```python
from build123d import *

# Parameters (mm, degrees)
F0_W     = 25.4
F0_H     = 6.35
F1_DEPTH = 6.35
F3_DEPTH = 25.4
F4_R     = 0.254
F5_R     = 0.254


with BuildPart() as f1:
    # F0 (on Top) → F1 (new body)
    with BuildSketch(Plane.XY):
        with Locations((12.7, 3.175)):
            Rectangle(F0_W, F0_H)
    extrude(amount=F1_DEPTH)

    # F2 (on face) → F3 (cut)
    with BuildSketch(Plane.XY.offset(6.35)):
        Polygon((15.621, 6.35), (12.7, 6.35), (14.1664696837, 3.81), (15.6269696837, 6.3396602045), align=None)
        Polygon((15.6329393675, 6.35), (15.621, 6.35), (15.6269696837, 6.3396602045), align=None)
        Polygon((15.6329393675, 6.35), (15.6269696837, 6.3396602045), (17.0874696837, 3.81), (18.5479696837, 6.3396602045), (18.542, 6.35), align=None)
        Polygon((18.5539393675, 6.35), (18.542, 6.35), (18.5479696837, 6.3396602045), align=None)
        Polygon((18.5539393675, 6.35), (18.5479696837, 6.3396602045), (20.0084696837, 3.81), (21.4689696837, 6.3396602045), (21.463, 6.35), align=None)
        Polygon((21.4749393675, 6.35), (21.463, 6.35), (21.4689696837, 6.3396602045), align=None)
        Polygon((21.4749393675, 6.35), (21.4689696837, 6.3396602045), (22.9294696837, 3.81), (24.3959393675, 6.35), align=None)
    extrude(amount=-F3_DEPTH, mode=Mode.SUBTRACT)

    # F4
    f4_edges = [f1.edges().sort_by_distance(p)[0] for p in [
        (21.46897, 6.33966, 3.175),
    ]]
    fillet(f4_edges, radius=F4_R)

    # F5
    f5_edges = [f1.edges().sort_by_distance(p)[0] for p in [
        (24.395939, 6.35, 3.175),
        (22.92947, 3.81, 3.175),
        (20.00847, 3.81, 3.175),
        (18.54797, 6.33966, 3.175),
        (17.08747, 3.81, 3.175),
        (15.62697, 6.33966, 3.175),
        (14.16647, 3.81, 3.175),
    ]]
    fillet(f5_edges, radius=F5_R)


solid = f1.part
```
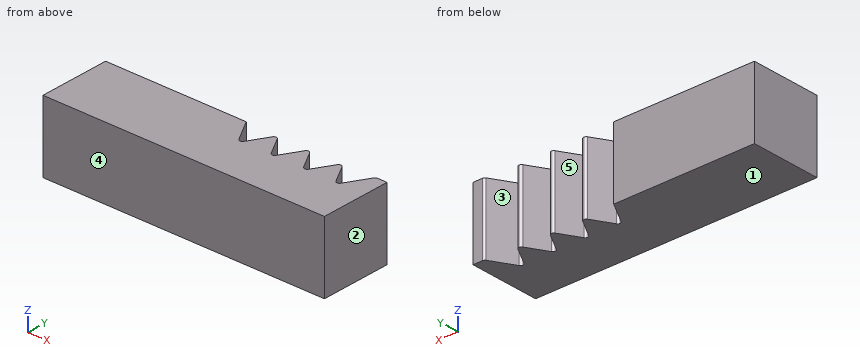
The listing builds one solid part. Answer for the finished solid, in the listing's coordinates (mm). Face numbers are marked on the shaded views. A direction names the side the tool comes from. Give positions to 0.01 mm unless a question says otherwise; leave off trailing zeros. Order: outer loops, then holes, each group sorted by start corner. A loop starts at its lowest first (then second) coordinate and runs counter-clockwise, first axis right, second up. Notation, with made-up numbers: (89, 62.25) -> (93, 62.25) arc R31 cw to (93, 97.25) -> close; hole circle Ø11 at (67, -31). An arc over 180 degrees is marked (long way). Answer as CSV lines item,"result". Start each with the question number.
Q1. Given pin 1 (1.5 mm diameter, centred on x = 2.5, y = 3, fed in from -Z), flat-ended and moving along its own axis, determine where the tip first touches the part or whether it passes through.
Q2. Which of the six approach directions +Z, -Z, +X, -X, +Y, -Y give full straight-line access (tool end or side, diameter ignored) to the marked faces 4 and 5?
Q3. A cutting plane is placed at C-C (x = 23.5). Determine the outline of the cut face in (y, z), then the cut area to 3 significant figures.
Q4. A cutting plane is placed at D-D (y = 4.5). Determine the outline of the cut face in (x, z).
Q5. Determine the mould class of the marked faces 1, 2 and 3 for opening direction X: pulls with the +X half, pulls with the -X half, needs draft (parallel to the pull), parting line crosses it, or undercut.
Q6. A cutting plane is placed at A-A (z = 1.5). Determine the outline of the cut face in (x, y).
Q7. A cutting plane is placed at B-B (y = 5.5). Determine the outline of the cut face in (x, z), then the cut area to 3 significant figures.
Q8. Find the intervals of material crossed by L1, parallel to X at y = 5, z = 1.75; L2, parallel to X at y = 5.25, z = 1.25; L3, parallel to X at y = 6.25, z = 5.5, in increasing order.
Results found:
1,pin 1,"z = 0"
2,face 4,"+Z, -Z, +X, -X, -Y"
2,face 5,"+Z, -Z, +Y"
3,outline,"(0, 0) -> (4.8, 0) -> (4.8, 6.35) -> (0, 6.35) -> close"
3,area,"30.5 mm2"
4,outline,"(0, 0) -> (13.77, 0) -> (13.77, 6.35) -> (0, 6.35) -> close; (14.56, 0) -> (16.69, 0) -> (16.69, 6.35) -> (14.56, 6.35) -> close; (17.49, 0) -> (19.61, 0) -> (19.61, 6.35) -> (17.49, 6.35) -> close; (20.41, 0) -> (22.53, 0) -> (22.53, 6.35) -> (20.41, 6.35) -> close; (23.33, 0) -> (25.4, 0) -> (25.4, 6.35) -> (23.33, 6.35) -> close"
5,face 1,"needs draft"
5,face 2,"pulls with the +X half"
5,face 3,"undercut"
6,outline,"(0, 0) -> (25.4, 0) -> (25.4, 6.35) -> (24.54, 6.35) arc R0.25 ccw to (24.32, 6.22) -> (23.15, 4.19) arc R0.25 cw to (22.71, 4.19) -> (21.69, 5.96) arc R0.25 ccw to (21.25, 5.96) -> (20.23, 4.19) arc R0.25 cw to (19.79, 4.19) -> (18.77, 5.96) arc R0.25 ccw to (18.33, 5.96) -> (17.31, 4.19) arc R0.25 cw to (16.87, 4.19) -> (15.85, 5.96) arc R0.25 ccw to (15.41, 5.96) -> (14.39, 4.19) arc R0.25 cw to (13.95, 4.19) -> (12.7, 6.35) -> (0, 6.35) -> close"
7,outline,"(0, 0) -> (13.19, 0) -> (13.19, 6.35) -> (0, 6.35) -> close; (15.14, 0) -> (16.11, 0) -> (16.11, 6.35) -> (15.14, 6.35) -> close; (18.06, 0) -> (19.03, 0) -> (19.03, 6.35) -> (18.06, 6.35) -> close; (20.98, 0) -> (21.95, 0) -> (21.95, 6.35) -> (20.98, 6.35) -> close; (23.91, 0) -> (25.4, 0) -> (25.4, 6.35) -> (23.91, 6.35) -> close"
7,area,"112 mm2"
8,L1,"0 to 13.48, 14.85 to 16.4, 17.77 to 19.32, 20.7 to 22.24, 23.62 to 25.4"
8,L2,"0 to 13.34, 15 to 16.26, 17.92 to 19.18, 20.84 to 22.1, 23.76 to 25.4"
8,L3,"0 to 12.76, 24.34 to 25.4"
